Verification items for the finished model (mm, model axes). A direction names the side the tool comes from. Round coordinates to 2 decimals unless told otherwise and drop trailing zeros. Loops run counter-clockwise (first coordinate to the right, second up) from the corner with the lowest first, then second, coordinate; pieces in that order, holes last. Notation, with made-up numbers: (-17.5, 63.5) - (30.5, 63.5) arc R16 cw to (30.5, 94.5) - close; hole circle Ø4 at (-22, -28.75). An arc over 180 degrees is marked (long way). Use a Markdown table: item, result. Add a question column.
```python
from build123d import *

# Parameters (mm, degrees)
F1_DEPTH = 6
F2_SIZE2 = 4
F2_SIZE  = 3.5
F3_DEPTH = 6
F4_DEPTH = 2


with BuildPart() as f1:
    # F0 (on Front) → F1 (new body)
    with BuildSketch(Plane.XZ):
        with BuildLine():
            Line((-17.2, 235), (-4.2, 235))
            Line((-4.2, 235), (-4.2, 241))
            Line((-4.2, 241), (-23.5591068412, 241))
            ThreePointArc((-23.5591068412, 241), (-47.1037067536, 126.5649280043), (-55, 10))
            Line((-55, 10), (-55, 0))
            Line((-55, 0), (-47, 0))
            Line((-47, 0), (-47, 10))
            ThreePointArc((-47, 10), (-45.6626874065, 58.0616713196), (-41.6548879545, 105.9746152759))
            Line((-41.6548879545, 105.9746152759), (-15.8, 105.9746152759))
            Line((-15.8, 105.9746152759), (-15.8, -9.5547260733))
            Line((-15.8, -9.5547260733), (-11.8, -9.5547260733))
            Line((-11.8, -9.5547260733), (-11.8, 197.0380991697))
            Line((-11.8, 197.0380991697), (-11.8, 202.0380991697))
            Line((-11.8, 202.0380991697), (-15.8, 202.0380991697))
            Line((-15.8, 202.0380991697), (-15.8, 197.0380991697))
            Line((-15.8, 197.0380991697), (-26.5197448355, 197.0380991697))
            ThreePointArc((-26.5197448355, 197.0380991697), (-22.0745066899, 216.0717428538), (-17.2, 235))
        make_face()
        with BuildLine():
            ThreePointArc((-41.198523154, 109.9746152759), (-35.3095909069, 151.6745341907), (-27.396421331, 193.0380991697))
            Line((-27.396421331, 193.0380991697), (-15.8, 193.0380991697))
            Line((-15.8, 193.0380991697), (-15.8, 109.9746152759))
            Line((-15.8, 109.9746152759), (-41.198523154, 109.9746152759))
        make_face(mode=Mode.SUBTRACT)
    extrude(amount=F1_DEPTH)

    # F2
    f2_edges = [f1.edges().sort_by_distance(p)[0] for p in [
        (-15.8, -3, -9.554726),
    ]]
    f2_side = f1.faces().sort_by_distance((-13.8, -3, -9.554726))[0]
    chamfer(f2_edges, length=F2_SIZE, length2=F2_SIZE2, reference=f2_side)

    # F3 (add): a face of the model
    f3_faces = [f1.faces().sort_by_distance(p)[0] for p in [
        (-47, -3, 5),
    ]]
    extrude(f3_faces, amount=F3_DEPTH)

    # F4 (cut): a face of the model
    f4_faces = [f1.faces().sort_by_distance(p)[0] for p in [
        (-44, -3, 10),
    ]]
    extrude(f4_faces, amount=-F4_DEPTH, mode=Mode.SUBTRACT)


solid = f1.part
```
Q1. Set-up check for faces 4 (the face through (-11.8, -3, 95)), 5 (the face through (-11, -3, 235)), 6 (the face through (-21, -3, 197.038)): record each of +Z, -Z, +X, -X, +Y, -Y from which the full face is reachable in a straight line by a thin tool's end or side.
Q2. Go/stop test with flat-tipped pins: pin 1 Ø1.8 at (x, y) = (-49.5, -3.5) entering from -Z; pin 2 Ø3 at (x, y) = (-13, -2.5) entering from -Z; pin 3 Ø1.6 at (y, z) = (-2, 8.5) entering from +X; pin 4 Ø3 at (x, y) = (-30.5, -2) entering from -Z. Record where each tip stops, or that it passes through.
Q3. Section check D-D on x = -30.5. Record the cut outline in (y, z), plus the area to 3 significant figures.
Q4. Release check for a two-part mould opening along X. For faces 1 (the face through (-43, 0, 115)), 2 (the face through (-15.8, -3, 51)), 3 (the face through (-14.1, -3, -7.5)) record: +X half, -X half, draft (parallel to the pull), parting line (faces both ways), or undercut.
Q5. Section check B-B on z = 85. Record the cut outline in (x, y).
Q6. Thickness scan on line 1 along Z through (x, y) = (-16.5, -2.3); line 2 along X through (y, z) = (-2.75, 9.5); line 3 along Z through (x, y) = (-10, -5.6). Record the ranges inside material, lowest first.
Q7. Section check C-C on x = -20. Record the cut outline in (y, z).
Q8. Section check A-A on y = -3.35. Record the cut outline in (x, z).
Determined:
| question | item | result |
|---|---|---|
| 1 | face 4 | -Z, +X, +Y, -Y |
| 1 | face 5 | +X, +Y, -Y |
| 1 | face 6 | +Y, -Y |
| 2 | pin 1 | stops at z = 0 |
| 2 | pin 2 | stops at z = -9.55 |
| 2 | pin 3 | stops at x = -11.8 |
| 2 | pin 4 | stops at z = 105.97 |
| 3 | outline | (-6, 105.97) - (0, 105.97) - (0, 109.97) - (-6, 109.97) - close; (-6, 178.08) - (0, 178.08) - (0, 214.33) - (-6, 214.33) - close |
| 3 | area | 242 mm² |
| 4 | face 1 | draft |
| 4 | face 2 | undercut |
| 4 | face 3 | -X half |
| 5 | outline | (-51.74, -6) - (-43.74, -6) - (-43.74, 0) - (-51.74, 0) - close; (-15.8, -6) - (-11.8, -6) - (-11.8, 0) - (-15.8, 0) - close |
| 6 | line 1 | z = 105.97 to 109.97, 193.04 to 197.04, 235 to 241 |
| 6 | line 2 | x = -55 to -47, -15.8 to -11.8 |
| 6 | line 3 | z = 235 to 241 |
| 7 | outline | (-6, 105.97) - (0, 105.97) - (0, 109.97) - (-6, 109.97) - close; (-6, 193.04) - (0, 193.04) - (0, 197.04) - (-6, 197.04) - close; (-6, 224.35) - (0, 224.35) - (0, 241) - (-6, 241) - close |
| 8 | outline | (-55, 0) - (-41, 0) - (-41, 8) - (-47, 8) - (-47, 10) arc R864.31 cw to (-41.65, 105.97) - (-15.8, 105.97) - (-15.8, -5.55) - (-12.3, -9.55) - (-11.8, -9.55) - (-11.8, 202.04) - (-15.8, 202.04) - (-15.8, 197.04) - (-26.52, 197.04) arc R864.31 cw to (-17.2, 235) - (-4.2, 235) - (-4.2, 241) - (-23.56, 241) arc R864.31 ccw to (-55, 10) - close; hole (-41.2, 109.97) - (-15.8, 109.97) - (-15.8, 193.04) - (-27.4, 193.04) arc R864.31 ccw to start |
